For this review, take the finished solid that the model builds, in its own axes (mm). A direction names the side the tool comes from. Give positions to 0.01 mm unless a question says otherwise; leave off trailing zeros. Order: outer loops, then holes, each group sorted by start corner. A loop starts at its lowest first (then second) coordinate and runs counter-clockwise, first axis right, second up. Notation, with made-up numbers: (78.5, 12.5) - (100.5, 12.5) arc R22 cw to (100.5, 41.5) - close; hole circle Ø5 at (-22, 3.5). An arc over 180 degrees is marked (long way). One line per item, written item: value.
```python
from build123d import *

# Parameters (mm, degrees)
F0_R        = 3.175
F1_DEPTH    = 6.35
F2_T1_DEPTH = 36.83
F3_T1_DEPTH = 36.83


# Not quite as in the source:
# - a fillet or chamfer that OpenCascade refuses, or shapes differently, is made with other operations: its cross-section is extruded or revolved along the edge and cut away or added


with BuildPart() as f1:
    # F0 (on Front) → F1 (new body)
    with BuildSketch(Plane.XZ):
        with BuildLine():
            Line((11.0398714598, -22.7022875817), (11.0398714598, 34.4477124183))
            Line((11.0398714598, 34.4477124183), (0, 34.4477124183))
            Line((0, 34.4477124183), (0, -11.9114368191))
            ThreePointArc((0, -11.9114368191), (-1.8598719395, -16.4015648796), (-6.35, -18.2614368191))
            Line((-6.35, -18.2614368191), (-33.4101285402, -18.2614368191))
            Line((-33.4101285402, -18.2614368191), (-33.4101285402, -29.0522875817))
            Line((-33.4101285402, -29.0522875817), (4.6898714598, -29.0522875817))
            ThreePointArc((4.6898714598, -29.0522875817), (9.1799995204, -27.1924156422), (11.0398714598, -22.7022875817))
        make_face()
        with Locations((-28.7397336215, -23.7723737955)):
            Circle(F0_R, mode=Mode.SUBTRACT)
        with Locations((4.6898714598, -22.7022875817)):
            Circle(F0_R, mode=Mode.SUBTRACT)
        with Locations((5.3221737035, 28.8079940212)):
            Circle(F0_R, mode=Mode.SUBTRACT)
    extrude(amount=F1_DEPTH)

    # F2: fillet of radius 6.096 on 2 edges, made by hand

    # F2_s2 → F2_t1 (cut)
    with BuildSketch(Plane.XZ.offset(-15.24)):
        with BuildLine():
            ThreePointArc((-27.3141285402, -18.2614368191), (-31.6246514783, -20.046913881), (-33.4101285402, -24.3574368191))
            Line((-33.4101285402, -24.3574368191), (-33.4101285402, -18.2614368191))
            Line((-33.4101285402, -18.2614368191), (-27.3141285402, -18.2614368191))
        make_face()
        with BuildLine():
            ThreePointArc((-33.4101285402, -22.9562875817), (-31.6246514783, -27.2668105198), (-27.3141285402, -29.0522875817))
            Line((-27.3141285402, -29.0522875817), (-33.4101285402, -29.0522875817))
            Line((-33.4101285402, -29.0522875817), (-33.4101285402, -22.9562875817))
        make_face()
    extrude(amount=F2_T1_DEPTH, mode=Mode.SUBTRACT)

    # F3: fillet of radius 6.096 on 2 edges, made by hand

    # F3_s2 → F3_t1 (cut)
    with BuildSketch(Plane.XZ.offset(-15.24)):
        with BuildLine():
            ThreePointArc((6.096, 34.4477124183), (1.7854770619, 32.6622353564), (0, 28.3517124183))
            Line((0, 28.3517124183), (0, 34.4477124183))
            Line((0, 34.4477124183), (6.096, 34.4477124183))
        make_face()
        with BuildLine():
            ThreePointArc((11.0398714598, 28.3517124183), (9.2543943979, 32.6622353564), (4.9438714598, 34.4477124183))
            Line((4.9438714598, 34.4477124183), (11.0398714598, 34.4477124183))
            Line((11.0398714598, 34.4477124183), (11.0398714598, 28.3517124183))
        make_face()
    extrude(amount=F3_T1_DEPTH, mode=Mode.SUBTRACT)


solid = f1.part
```
(1) Wall thickness on line 1 (X direction, y = -1.5, z = 22); line 2 (Z direction, x = -7, y = -3.5); line 3 (Z direction, x = 2.5, y = -1.5): over which ranges is each line inside the solid? List them lowest first. Write a range as from..to.
Answers below:
line 1: x = 0..11.04
line 2: z = -29.05..-18.26
line 3: z = -29.05..-25, -20.4..27.35, 30.26..33.27
(2) Take a section at B-B (x = -21.5). Write out the cut boundary in (y, z), then the cut area to 3 significant figures.
Answers below:
outline: (-6.35, -29.05) - (0, -29.05) - (0, -18.26) - (-6.35, -18.26) - close
area: 68.5 mm^2
(3) Take a section at C-C (z = 6). Write out the cut boundary in (x, y), then the cut area to 3 significant figures.
Answers below:
outline: (0, -6.35) - (11.04, -6.35) - (11.04, 0) - (0, 0) - close
area: 70.1 mm^2
(4) Take a section at A-A (y = -3). Write out the cut boundary in (x, z) (3 decimals), then the cut area to 3 significant figures.
Answers below:
outline: (-33.37, -23.657) arc R6.096 ccw to (-27.314, -29.052) - (4.69, -29.052) arc R6.35 ccw to (11.04, -22.702) - (11.04, 28.352) arc R6.096 ccw to (5.52, 34.42) arc R6.096 ccw to (0, 28.352) - (0, -11.911) arc R6.35 cw to (-6.35, -18.261) - (-27.314, -18.261) arc R6.096 ccw to start; hole circle Ø6.35 at (-28.74, -23.772); hole circle Ø6.35 at (4.69, -22.702); hole circle Ø6.35 at (5.322, 28.808)
area: 935 mm^2
(5) Draft analysis for pull direction Z (two halves, no side actions). For faces 1 (the face through (0.2, 0, -8.9)), 2 (the face through (2.17, -3.131, -24.634)), 3 (the face through (-31.416, -3.131, -27.466)), 4 (the face through (-1.81, -3.13, -16.35)), state which applies: pulls with the +Z half, pulls with the -Z half, needs draft (parallel to the pull), parting line crosses it, or undercut.
Answers below:
face 1: needs draft
face 2: undercut
face 3: pulls with the -Z half
face 4: pulls with the +Z half
(6) For P1, Ø6, axis at x = -15.5, z = -14.5, coming from the +Y side; P2, Ø3, axis at y = -1.5, z = -20, coming from the -X side, all flat-tipped, find the tip position at first contact; note any pin that passes through.
Answers below:
P1: passes through
P2: stops at x = -32.7
(7) Machinability: for faces 5 (the face through (4.909, -3.131, 31.956)), 6 (the face through (-17, -3, -18.261)), which of the approach directions +Z, -Z, +X, -X, +Y, -Y give a long, thin tool a straight path to every point of the face, cutting with its end or side? Answer none if there is none.
Answers below:
face 5: +Y, -Y
face 6: +Z, -X, +Y, -Y
